Can you work these out from the model? Positions are in its coordinate system, mm. Face numbers are marked on the shaded views. A direction names the side the tool comes from. Round coordinates to 2 decimals unless told otherwise and drop trailing zeros. Order: outer loops, then holes, each group sorted by start corner. A loop starts at its lowest first (then second) coordinate and runs counter-clockwise, first axis right, second up. Notation, with made-up numbers: (85, 34.25) - (128, 34.25) arc R20 ccw to (128, 61.25) - close; hole circle Ø4 at (-17, 28.25). An arc over 180 degrees is marked (long way). Write item = value, one per line.
from build123d import *

# Parameters (mm, degrees)
SKETCH1_R           = 5.5
SKETCH1_R_2         = 5
BOSS_EXTRUDE1_DEPTH = 10
SKETCH1_3_R         = 5.5
SKETCH1_3_R_2       = 5
BOSS_EXTRUDE2_DEPTH = 80
BOSS_EXTRUDE3_START = -10
SKETCH2_R           = 5.5
SKETCH2_R_2         = 5
BOSS_EXTRUDE3_DEPTH = 10


with BuildPart() as part:
    # Sketch1 → Boss-Extrude1 (new body)
    with BuildSketch(Plane.XY):
        with BuildLine():
            Line((0, 10), (0, 50))
            ThreePointArc((0, 50), (10, 60), (20, 50))
            Line((20, 50), (20, 10))
            ThreePointArc((20, 10), (10, 0), (0, 10))
        make_face()
        with Locations((10, 50)):
            Circle(SKETCH1_R, mode=Mode.SUBTRACT)
        with Locations((10, 10)):
            Circle(SKETCH1_R_2, mode=Mode.SUBTRACT)
    extrude(amount=BOSS_EXTRUDE1_DEPTH)

    # Sketch1_3 → Boss-Extrude2 (add)
    with BuildSketch(Plane.XY):
        with Locations((10, 50)):
            Circle(SKETCH1_3_R)
        with Locations((10, 50)):
            Circle(SKETCH1_3_R_2, mode=Mode.SUBTRACT)
    extrude(amount=BOSS_EXTRUDE2_DEPTH)

    # Sketch2 → Boss-Extrude3 (add)
    with BuildSketch(Plane.XY.offset(80).offset(BOSS_EXTRUDE3_START)):
        with BuildLine():
            Line((20, 90), (20, 50))
            ThreePointArc((20, 50), (10, 40), (0, 50))
            Line((0, 50), (0, 90))
            ThreePointArc((0, 90), (10, 100), (20, 90))
        make_face()
        with Locations((10, 50)):
            Circle(SKETCH2_R, mode=Mode.SUBTRACT)
        with Locations((10, 90)):
            Circle(SKETCH2_R_2, mode=Mode.SUBTRACT)
    extrude(amount=BOSS_EXTRUDE3_DEPTH)


solid = part.part
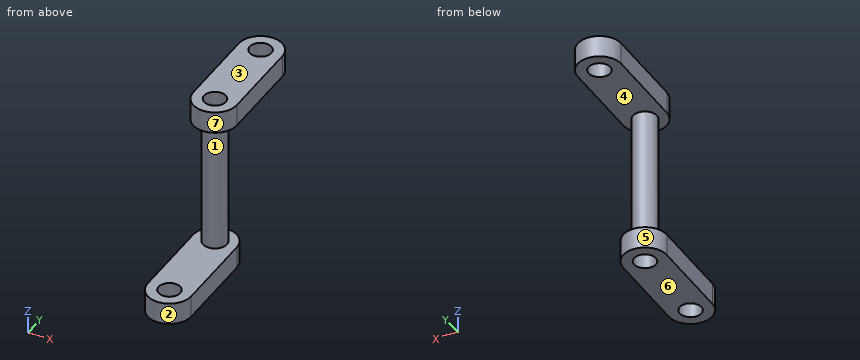
(1) Will these pins go through, and if not, where does the flat tip stop? P1, Ø9, axis at x = 10, y = 10, coming from the -Z side; P2, Ø10, axis at x = 8, z = 54, coming from the +Y side; P3, Ø10, axis at x = 9.5, y = 16, coming from the +Z side; P4, Ø1, axis at x = 13.5, z = 52, coming from the +Y side.
Computed:
P1 = through
P2 = 55.5
P3 = 10
P4 = 54.61
(2) If we section it at C-C (z = 63): Write out the boundary of the cut face in (x, y), plus the area to 3 significant figures.
Computed:
outline = circle Ø11 at (10, 50); hole circle Ø10 at (10, 50)
area = 16.5 mm^2
(3) Thinking about a two-plate mould opening in Z: for the marked faces 1, 2, 3 and 4, which applies, +Z half, -Z half, draft (parallel to the pull), parting line (faces both ways), or undercut?
Computed:
face_1 = undercut
face_2 = draft
face_3 = +Z half
face_4 = undercut
(4) On a 3-axis mill with a long thin cutter (end or side, diameter ignored), from which of +Z, -Z, +X, -X, +Y, -Y can I reach the whole of each face in a straight line? I mean the marked faces 5, 6 and 7. Say none if no direction works.
Computed:
face_5 = -Z, +Y
face_6 = -Z, +X, -X, +Y, -Y
face_7 = +Z, -Y
(5) If we section it at B-B (x = 10): Write out the boundary of the cut face in (y, z), plus the area to 3 significant figures.
Computed:
outline = (0, 0) - (5, 0) - (5, 10) - (0, 10) - close; (15, 0) - (45, 0) - (45, 80) - (40, 80) - (40, 70) - (44.5, 70) - (44.5, 10) - (15, 10) - close; (55, 0) - (60, 0) - (60, 10) - (55.5, 10) - (55.5, 70) - (85, 70) - (85, 80) - (55, 80) - close; (95, 70) - (100, 70) - (100, 80) - (95, 80) - close
area = 860 mm^2
(6) If I drill on line 1 (Y direction, x = 10, z = 7); line 2 (Y direction, x = 10, z = 77.75); line 3 (Z direction, x = 16.5, y = 47), over which ranges is the centre line in solid material (lowest first)? Write a range as from..to.
Computed:
line_1 = 0..5, 15..45, 55..60
line_2 = 40..45, 55..85, 95..100
line_3 = 0..10, 70..80
(7) If we section it at A-A (y = 13): Write out the boundary of the cut face in (x, z), plus the area to 3 significant figures.
Computed:
outline = (0, 0) - (6, 0) - (6, 10) - (0, 10) - close; (14, 0) - (20, 0) - (20, 10) - (14, 10) - close
area = 120 mm^2
(8) If we section it at D-D (y = 58): Write out the boundary of the cut face in (x, z), plus the area to 3 significant figures.
Computed:
outline = (0, 70) - (20, 70) - (20, 80) - (0, 80) - close; (4, 0) - (16, 0) - (16, 10) - (4, 10) - close
area = 320 mm^2
